Part model, mm, in its own coordinate system. Face numbers are marked on the shaded views. A direction names the side the tool comes from. Give positions to 0.01 mm unless a question says otherwise; leave off trailing zeros. Write each loop counter-clockwise with the first axis right and the second up, starting at its lowest first coordinate (ties: lowest second). Pieces come first, ordered by that corner, then holes. Notation, with made-up numbers: M 1,86.5 L 30,86.5 A24 cw 30,107.5 Z; hole C 5.25,-22.75 d7. An arc over 180 degrees is marked long. Write item = value, one per line. Start each with the question number.
from build123d import *

# Parameters (mm, degrees)
SKETCH1_W   = 7.5
SKETCH1_H   = 20
SKETCH1_W_2 = 6
SKETCH1_H_2 = 12
SKETCH1_W_3 = 2.5
SKETCH1_H_3 = 5
FILLET1_R   = 1


with BuildPart() as part:
    # Sketch1 → Revolve1 (revolve)
    with BuildSketch(Plane.XY):
        with Locations((-3.75, -10)):
            Rectangle(SKETCH1_W, SKETCH1_H)
        with Locations((-3, 6)):
            Rectangle(SKETCH1_W_2, SKETCH1_H_2)
        Polygon((-6, 12), (0, 12), (0, 16.2), (-2.5, 16.2), (-7.5, 16.2), (-7.5, 12), align=None)
        with Locations((-1.25, 18.7)):
            Rectangle(SKETCH1_W_3, SKETCH1_H_3)
    revolve(axis=Axis((0, 25.269315462, 0), (0, -1, 0)))

    # Fillet1
    fillet1_edges = [part.edges().sort_by_distance(p)[0] for p in [
        (6, 0, 0),
        (6, 12, 0),
    ]]
    fillet(fillet1_edges, radius=FILLET1_R)


solid = part.part
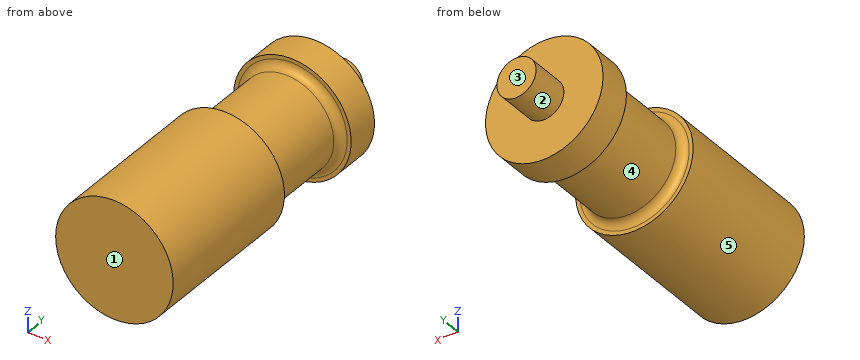
Q1. Drop flat-ended pins along their axis: P1, Ø5, axis at y = 1, z = -4.5, coming from the -X side; P2, Ø6, axis at x = -3, z = 5.5, coming from the +Y side; P3, Ø8, axis at x = -4.5, z = -2.5, coming from the +Y side; P4, Ø2, axis at x = 1.5, y = -3.5, coming from the +Z side. Give the stop position or say it passes through.
Q2. Slice it at B-B (x = 0). Give the cut face in (y, z).
Q3. Probe line 1 along Y through (x, z) = (5.5, -0.5); line 2 along Y through (x, z) = (-6.25, 0); line 3 along Z through (x, y) = (-2, -13.5). List the from-to ranges inside material, lowest first.
Q4. Tool access for the marked faces 1 and 2: list every direction of +Z, -Z, +X, -X, +Y, -Y with a clear straight run to the whole face (end or side of a thin tool).
Q5. Slice it at C-C (y = 8.5). Give the cut face in (x, z).
Q6. Slice it at D-D (y = 17). Give the cut face in (x, z).
Q7. Slice it at A-A (z = 0). Give the cut face in (x, y), and give its area (3 significant figures).
Q8. Two-plate mould, pull along Y, no slides. Class the marked faces 3, 4 and 5: +Y half, -Y half, draft (parallel to the pull), parting line (faces both ways), or undercut.
Working result:
q1.P1 = -7.17
q1.P2 = 16.2
q1.P3 = 21.2
q1.P4 = 7.48
q2.outline = M -20,-7.5 L 0,-7.5 L 0,-7 A1 cw 1,-6 L 11,-6 A1 cw 12,-7 L 12,-7.5 L 16.2,-7.5 L 16.2,-2.5 L 21.2,-2.5 L 21.2,2.5 L 16.2,2.5 L 16.2,7.5 L 12,7.5 L 12,7 A1 cw 11,6 L 1,6 A1 cw 0,7 L 0,7.5 L -20,7.5 Z
q3.line_1 = -20 to 16.2
q3.line_2 = -20 to 0.34, 11.66 to 16.2
q3.line_3 = -7.23 to 7.23
q4.face_1 = +Z, -Z, +X, -X, -Y
q4.face_2 = +Y
q5.outline = C 0,0 d12
q6.outline = C 0,0 d5
q7.outline = M -7.5,-20 L 7.5,-20 L 7.5,0 L 7,0 A1 cw 6,1 L 6,11 A1 cw 7,12 L 7.5,12 L 7.5,16.2 L 2.5,16.2 L 2.5,21.2 L -2.5,21.2 L -2.5,16.2 L -7.5,16.2 L -7.5,12 L -7,12 A1 cw -6,11 L -6,1 A1 cw -7,0 L -7.5,0 Z
q7.area = 533 mm2
q8.face_3 = +Y half
q8.face_4 = undercut
q8.face_5 = draft
